Source: CAD feature listing. Evaluate the final solid. Frame: model axes, mm. Face numbers are marked on the shaded views. A direction names the side the tool comes from. Round coordinates to 2 decimals unless told otherwise and drop trailing zeros. Order: outer loops, then holes, each group sorted by start corner. A loop starts at its lowest first (then second) coordinate and runs counter-clockwise, first axis right, second up. Notation, with made-up numbers: (8, 80.5) -> (54, 80.5) arc R27 ccw to (54, 119.5) -> close; hole circle Ø9 at (89.5, -14). An arc over 180 degrees is marked (long way). Answer as CSV lines item,"result".
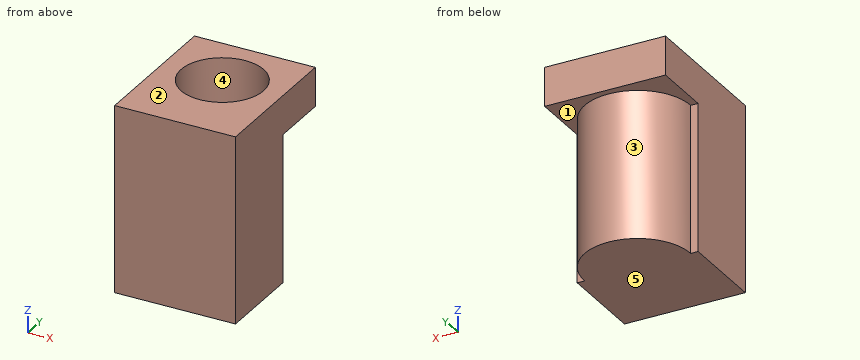
from build123d import *

# Parameters (mm, degrees)
SKETCH1_W           = 9
SKETCH1_H           = 10.9
BOSS_EXTRUDE1_DEPTH = 2.9
BOSS_EXTRUDE2_DEPTH = 11
SKETCH3_R           = 3.075
CUT_EXTRUDE1_DEPTH  = 9


with BuildPart() as part:
    # Sketch1 → Boss-Extrude1 (new body)
    with BuildSketch(Plane.XY):
        Rectangle(SKETCH1_W, SKETCH1_H)
    extrude(amount=BOSS_EXTRUDE1_DEPTH)

    # Sketch2 → Boss-Extrude2 (add)
    with BuildSketch(Plane(origin=(0, 0, 0), x_dir=(-1, 0, 0), z_dir=(0, 0, -1))):
        with BuildLine():
            Line((-3.95, 1), (-4.5, 1))
            Line((-4.5, 1), (-4.5, -5.45))
            Line((-4.5, -5.45), (4.5, -5.45))
            Line((4.5, -5.45), (4.5, 1))
            Line((4.5, 1), (3.95, 1))
            ThreePointArc((3.95, 1), (0, 4.95), (-3.95, 1))
        make_face()
    extrude(amount=BOSS_EXTRUDE2_DEPTH)

    # Sketch3 → Cut-Extrude1 (cut)
    with BuildSketch(Plane.XY.offset(2.9)):
        with Locations((0, 1)):
            Circle(SKETCH3_R)
    extrude(amount=-CUT_EXTRUDE1_DEPTH, mode=Mode.SUBTRACT)


solid = part.part
1. Section query C-C on y = 1.25. Return loops of the section in (x, z), and give its area (3 significant figures).
Results below:
outline,"(-4.5, 0) -> (-3.94, 0) -> (-3.94, -11) -> (3.94, -11) -> (3.94, 0) -> (4.5, 0) -> (4.5, 2.9) -> (3.06, 2.9) -> (3.06, -6.1) -> (-3.06, -6.1) -> (-3.06, 2.9) -> (-4.5, 2.9) -> close"
area,"57.7 mm2"
2. Reachability of the marked faces 1 and 2 from +Z, -Z, +X, -X, +Y, -Y: full face, straight path, thin tool, end or side. Return the list, or none.
Results below:
face 1,"-Z, +Y"
face 2,"+Z, +X, -X, +Y, -Y"
3. Line query: L1, parallel to Y at x = 0, z = -4 (3 decimals); L2, parallel to Y at x = 0, z = 0.5 (3 decimals); L3, parallel to Z at x = 2.5, y = 2. Output: solid intervals per line, ascending. Write a range as [from, to].
Results below:
L1,"[-5.45, -2.075], [4.075, 4.95]"
L2,"[-5.45, -2.075], [4.075, 5.45]"
L3,"[-11, -6.1]"
4. Section query A-A on z = -1. Return loops of the section in (x, y) (3 decimals), and give its area (3 significant figures).
Results below:
outline,"(-4.5, -5.45) -> (4.5, -5.45) -> (4.5, 1) -> (3.95, 1) arc R3.95 ccw to (-3.95, 1) -> (-4.5, 1) -> close; hole circle Ø6.15 at (0, 1)"
area,"52.9 mm2"
5. Pin query (flat end, axial travel): pin 1 (1.5 mm diameter, centred on x = -1.5, y = 1, fed in from +Z); pin 2 (0.6 mm diameter, centred on x = -4.5, z = -3.5, fed in from +Y); pin 3 (2 mm diameter, centred on y = 4, z = -2.5, fed in from +X). Return the tip coordinate at first contact, or that it passes through.
Results below:
pin 1,"z = -6.1"
pin 2,"y = 1"
pin 3,"x = 3.41"
6. Mould query, pull axis X, two halves, no side actions, for the marked faces 3, 4 and 5. Classes: released by +X, released by -X, zero draft, split by the parting line, or undercut.
Results below:
face 3,"split by the parting line"
face 4,"undercut"
face 5,"zero draft"
7. Section query B-B on x = 0. Return loops of the section in (y, z) (3 decimals).
Results below:
outline,"(-5.45, -11) -> (4.95, -11) -> (4.95, 0) -> (5.45, 0) -> (5.45, 2.9) -> (4.075, 2.9) -> (4.075, -6.1) -> (-2.075, -6.1) -> (-2.075, 2.9) -> (-5.45, 2.9) -> close"
8. Section query D-D on x = 1.75. Return loops of the section in (y, z), and give its area (3 significant figures).
Results below:
outline,"(-5.45, -11) -> (4.54, -11) -> (4.54, 0) -> (5.45, 0) -> (5.45, 2.9) -> (3.53, 2.9) -> (3.53, -6.1) -> (-1.53, -6.1) -> (-1.53, 2.9) -> (-5.45, 2.9) -> close"
area,"96.0 mm2"
